Build history of the part. All positions in model axes, mm. Round coordinates to 2 decimals unless told otherwise and drop trailing zeros. Loops run counter-clockwise (first coordinate to the right, second up) from the corner with the lowest first, then second, coordinate; pieces in that order, holes last. Notation, with made-up numbers: M 34.25,66.25 L 61.25,66.25 A35 ccw 61.25,98.25 Z; hole C 16,-14.5 d9. An arc over 180 degrees is marked long. One line per item, written item: value.
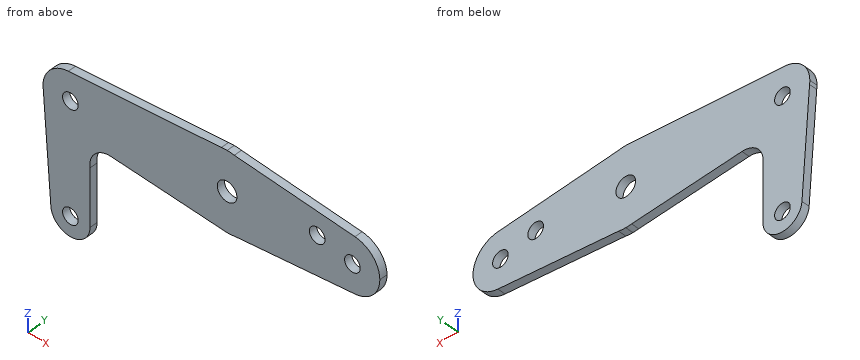
```python
from build123d import *

# Parameters (mm, degrees)
F0_R     = 3.9751
F0_R_2   = 3.175
F1_DEPTH = 3.175


with BuildPart() as f1:
    # F0 (on Front) → F1 (new body)
    with BuildSketch(Plane.XZ):
        with BuildLine():
            ThreePointArc((2.9215490166, -15.6038513305), (12.2146472655, -10.1399219514), (15.875, 0))
            ThreePointArc((15.875, 0), (12.2146472655, 10.1399219514), (2.9215490166, 15.6038513305))
            Line((2.9215490166, 15.6038513305), (0, 15.875))
            Line((0, 15.875), (-2.3527821949, 15.6996828294))
            ThreePointArc((-2.3527821949, 15.6996828294), (-15.875, 0), (-2.3527821949, -15.6996828294))
            Line((-2.3527821949, -15.6996828294), (0, -15.875))
            Line((0, -15.875), (2.9215490166, -15.6038513305))
        make_face()
        Circle(F0_R, mode=Mode.SUBTRACT)
        with BuildLine():
            ThreePointArc((2.9215490166, 15.6038513305), (12.2146472655, 10.1399219514), (15.875, 0))
            ThreePointArc((15.875, 0), (12.2146472655, -10.1399219514), (2.9215490166, -15.6038513305))
            Line((2.9215490166, -15.6038513305), (51.8269366371, -11.0649472386))
            ThreePointArc((51.8269366371, -11.0649472386), (39.6875, 0), (51.8269366371, 11.0649472386))
            Line((51.8269366371, 11.0649472386), (2.9215490166, 15.6038513305))
        make_face()
        with Locations((36.5252, 3.175)):
            Circle(F0_R_2, mode=Mode.SUBTRACT)
        with BuildLine():
            Line((0, 15.875), (2.9215490166, 15.6038513305))
            ThreePointArc((2.9215490166, 15.6038513305), (1.4670523387, 15.8070674837), (0, 15.875))
        make_face()
        with BuildLine():
            ThreePointArc((0, -15.875), (1.4670523387, -15.8070674837), (2.9215490166, -15.6038513305))
            Line((2.9215490166, -15.6038513305), (0, -15.875))
        make_face()
        with BuildLine():
            Line((-2.3527821949, 15.6996828294), (0, 15.875))
            ThreePointArc((0, 15.875), (-1.1796525089, 15.8311100356), (-2.3527821949, 15.6996828294))
        make_face()
        with BuildLine():
            ThreePointArc((61.9125, 0), (59.0127793599, 7.4858474093), (51.8269366371, 11.0649472386))
            ThreePointArc((51.8269366371, 11.0649472386), (39.6875, 0), (51.8269366371, -11.0649472386))
            ThreePointArc((51.8269366371, -11.0649472386), (59.0127793599, -7.4858474093), (61.9125, 0))
        make_face()
        with Locations((50.8, 0)):
            Circle(F0_R_2, mode=Mode.SUBTRACT)
        with BuildLine():
            ThreePointArc((-2.3527821949, -15.6996828294), (-1.1796525089, -15.8311100356), (0, -15.875))
            Line((0, -15.875), (-2.3527821949, -15.6996828294))
        make_face()
        with BuildLine():
            ThreePointArc((-2.3527821949, -15.6996828294), (-15.875, 0), (-2.3527821949, 15.6996828294))
            Line((-2.3527821949, 15.6996828294), (-64.3257567562, 11.0817770249))
            ThreePointArc((-64.3257567562, 11.0817770249), (-55.9398599783, 8.1444422216), (-52.3875, 0))
            ThreePointArc((-52.3875, 0), (-62.7132218511, -11.0846125956), (-74.5010903522, -1.5696073753))
            Line((-74.5010903522, -1.5696073753), (-71.4175804254, -45.0119843921))
            ThreePointArc((-71.4175804254, -45.0119843921), (-63.7811686533, -36.5174814568), (-55.5625, -44.45))
            Line((-55.5625, -44.45), (-55.5625, -21.4296542108))
            ThreePointArc((-55.5625, -21.4296542108), (-53.5062463335, -14.8690750057), (-47.1031557359, -12.3651162511))
            Line((-47.1031557359, -12.3651162511), (-2.3527821949, -15.6996828294))
        make_face()
        with BuildLine():
            ThreePointArc((-52.3875, 0), (-55.9398599783, 8.1444422216), (-64.3257567562, 11.0817770249))
            ThreePointArc((-64.3257567562, 11.0817770249), (-71.6444422216, 7.5601400217), (-74.6125, 0))
            Line((-74.6125, 0), (-74.5010903522, -1.5696073753))
            ThreePointArc((-74.5010903522, -1.5696073753), (-62.7132218511, -11.0846125956), (-52.3875, 0))
        make_face()
        with Locations((-63.5, 0)):
            Circle(F0_R_2, mode=Mode.SUBTRACT)
        with BuildLine():
            Line((-74.5010903522, -1.5696073753), (-74.6125, 0))
            ThreePointArc((-74.6125, 0), (-74.5846125956, -0.7867781489), (-74.5010903522, -1.5696073753))
        make_face()
        with BuildLine():
            ThreePointArc((-71.4175804254, -45.0119843921), (-63.2188313467, -52.3825185432), (-55.5625, -44.45))
            ThreePointArc((-55.5625, -44.45), (-63.7811686533, -36.5174814568), (-71.4175804254, -45.0119843921))
        make_face()
        with Locations((-63.5, -44.45)):
            Circle(F0_R_2, mode=Mode.SUBTRACT)
    extrude(amount=F1_DEPTH)


solid = f1.part
```
Item 1: Slice it at C-C, the plane x = -8. Give the cut face in (y, z) (3 decimals), and give its area (3 significant figures).
Check values:
outline: M -3.175,-15.279 L 0,-15.279 L 0,15.279 L -3.175,15.279 Z
area: 97.0 mm2
Item 2: Slice it at A-A, the plane y = -1.2. Give the number of separate pieces and of enclosed holes in the cut face, and give its area (3 significant figures).
Check values:
separate pieces: 1
enclosed holes: 5
area: 4,000 mm2
Item 3: Slice it at B-B, the plane z = -42.5. Give the cut face in (x, y) (1 decimal), and give its area (3 significant figures).
Check values:
outline: M -71.6,-3.2 L -66,-3.2 L -66,0 L -71.6,0 Z; M -61,-3.2 L -55.6,-3.2 L -55.6,0 L -61,0 Z
area: 35.0 mm2
Item 4: Slice it at D-D, the plane x = 20. Give the cut face in (y, z) (3 decimals).
Check values:
outline: M -3.175,-14.019 L 0,-14.019 L 0,14.019 L -3.175,14.019 Z
Item 5: Wall check: line 1 along Z through (x, y) = (-63.5, -2.15) (1 decimal); line 2 along X through (y, z) = (-1.8, 2.5); line 3 along Z through (x, y) = (0, -1.85) (3 decimals). Give the ranges that are in metal, low to high.
Check values:
line 1: z = -52.4 to -47.6, -41.3 to -3.2, 3.2 to 11.1
line 2: x = -74.33 to -65.46, -61.54 to -3.09, 3.09 to 33.42, 39.63 to 48.84, 52.76 to 61.63
line 3: z = -15.875 to -3.975, 3.975 to 15.875
Item 6: Drop flat-ended pins along their axis: P1, Ø7.5, axis at x = 36.53, z = 3.18, coming from the -Y side (3 decimals); P2, Ø1, axis at y = -1.5, z = -28.5, coming from the +X side. Give the stop position or say it passes through.
Check values:
P1: stops at y = -3.175
P2: stops at x = -55.56
